Input: part model. Units: mm. Frame: model coordinates. Face numbers are marked on the shaded views. A direction names the side the tool comes from. Give positions to 0.01 mm unless a question says otherwise; leave off trailing zeros. Write each loop counter-clockwise with the first axis right and the second up, starting at its lowest first coordinate (ties: lowest second). Pieces come first, ordered by that corner, then holes.
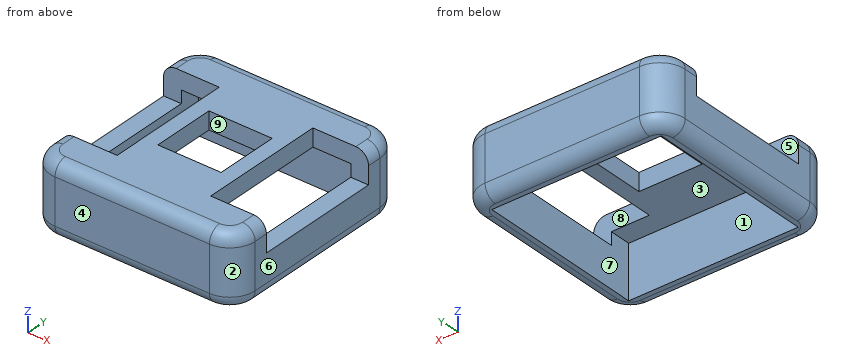
```python
from build123d import *

# Parameters (mm, degrees)
F0_W      = 20.574
F0_H      = 20.574
F1_DEPTH  = 7.112
F2_W      = 17.018
F2_H      = 17.018
F3_DEPTH  = 5.334
F4_R      = 2.54
F5_W      = 5.588
F5_H      = 12.7
F6_DEPTH  = 3.048
F7_W      = 11.176
F7_H      = 12.7
F8_DEPTH  = 3.048
F9_W      = 6.35
F9_H      = 6.35
F10_DEPTH = 1.778
F11_R     = 1.27
F12_R     = 1.27


with BuildPart() as f1:
    # F0 (on Top) → F1 (new body)
    with BuildSketch(Plane.XY):
        Rectangle(F0_W, F0_H)
    extrude(amount=F1_DEPTH)

    # F2 (on face) → F3 (cut)
    with BuildSketch(Plane(origin=(0, 0, 0), x_dir=(1, 0, 0), z_dir=(0, 0, -1))):
        Rectangle(F2_W, F2_H)
    extrude(amount=-F3_DEPTH, mode=Mode.SUBTRACT)

    # F4
    f4_edges = [f1.edges().sort_by_distance(p)[0] for p in [
        (-10.287, -10.287, 3.556),
        (10.287, 10.287, 3.556),
        (10.287, -10.287, 3.556),
        (-10.287, 10.287, 3.556),
    ]]
    fillet(f4_edges, radius=F4_R)

    # F5 (on face) → F6 (cut)
    with BuildSketch(Plane.XY.offset(7.112)):
        with Locations((-7.493, 0)):
            Rectangle(F5_W, F5_H)
    extrude(amount=-F6_DEPTH, mode=Mode.SUBTRACT)

    # F7 (on face) → F8 (cut)
    with BuildSketch(Plane.XY.offset(7.112)):
        with Locations((10.287, 0)):
            Rectangle(F7_W, F7_H)
    extrude(amount=-F8_DEPTH, mode=Mode.SUBTRACT)

    # F9 (on face) → F10 (cut)
    with BuildSketch(Plane.XY.offset(7.112)):
        Rectangle(F9_W, F9_H)
    extrude(amount=-F10_DEPTH, mode=Mode.SUBTRACT)

    # F11
    f11_edges = [f1.edges().sort_by_distance(p)[0] for p in [
        (0, 10.287, 7.112),
        (0, -10.287, 7.112),
    ]]
    fillet(f11_edges, radius=F11_R)

    # F12
    f12_edges = [f1.edges().sort_by_distance(p)[0] for p in [
        (-10.287, 0, 0),
        (0, 10.287, 0),
        (-9.543051, 9.543051, 0),
    ]]
    fillet(f12_edges, radius=F12_R)


solid = f1.part
```
Item 1: Section C-C (x = -7.5). Return loops of the section in (y, z).
Item 2: Section D-D (y = -5.75). Return loops of the section in (x, z).
Item 3: Pin query (flat end, axial travel): pin 1 (2 mm diameter, centred on x = -10, y = 2.5, fed in from +Z); pin 2 (1.5 mm diameter, centred on x = 0, z = 6.5, fed in from +Y); pin 3 (0.5 mm diameter, centred on y = -1, z = 6.5, fed in from +X); pin 4 (2 mm diameter, centred on y = 0.5, z = 6.5, fed in from -X). Return the tip coordinate at first contact, or that it passes through.
Item 4: Mould query, pull axis X, two halves, no side actions, for the marked faces 1, 2, 3 and 4. Classes: +X half, -X half, draft (parallel to the pull), parting line (faces both ways), or undercut.
Item 5: Set-up query: the marked faces 5, 6, 7, 8 and 9. Return all of +Z, -Z, +X, -X, +Y, -Y with unobstructed straight access to the full face (end or side cutting, diameter ignored); none if empty.
Item 6: Ray query, line 1 (Y direction, x = -4, z = 5); line 2 (Y direction, x = -4.75, z = 5.5). Return the intervals inside material, ascending.
Item 7: Section B-B (z = 4.75). Return loops of the section in (x, y), and give its area (3 significant figures).
Item 8: Section A-A (y = 2.5). Return loops of the section in (x, z) (3 decimals), and give its area (3 significant figures).
Solved:
1. outline: (-10.29, 1.27) arc R1.27 ccw to (-9.02, 0) - (-8.51, 0) - (-8.51, 5.33) - (-6.35, 5.33) - (-6.35, 7.11) - (-9.02, 7.11) arc R1.27 ccw to (-10.29, 5.84) - close; (6.35, 5.33) - (8.51, 5.33) - (8.51, 0) - (9.02, 0) arc R1.27 ccw to (10.29, 1.27) - (10.29, 5.84) arc R1.27 ccw to (9.02, 7.11) - (6.35, 7.11) - close
2. outline: (-10.29, 1.27) arc R1.27 ccw to (-9.02, 0) - (-8.51, 0) - (-8.51, 4.06) - (-10.29, 4.06) - close; (-4.7, 5.33) - (4.7, 5.33) - (4.7, 7.11) - (-4.7, 7.11) - close; (8.51, 0) - (9.02, 0) arc R1.27 ccw to (10.29, 1.27) - (10.29, 4.06) - (8.51, 4.06) - close
3. pin 1: stops at z = 4.06
3. pin 2: stops at y = 10.29
3. pin 3: stops at x = 4.7
3. pin 4: stops at x = -4.7
4. face 1: undercut
4. face 2: +X half
4. face 3: undercut
4. face 4: draft
5. face 5: +Z, -X
5. face 6: +Z, -Z, +X, +Y, -Y
5. face 7: -Z
5. face 8: +Z, +X
5. face 9: +Z, -Z
6. line 1: y = -10.29 to -8.51, 8.51 to 10.29
6. line 2: y = -10.29 to -6.35, 6.35 to 10.29
7. outline: (-10.29, -7.75) arc R2.54 ccw to (-7.75, -10.29) - (7.75, -10.29) arc R2.54 ccw to (10.29, -7.75) - (10.29, -6.35) - (8.51, -6.35) - (8.51, -8.51) - (-8.51, -8.51) - (-8.51, -6.35) - (-10.29, -6.35) - close; (-10.29, 6.35) - (-8.51, 6.35) - (-8.51, 8.51) - (8.51, 8.51) - (8.51, 6.35) - (10.29, 6.35) - (10.29, 7.75) arc R2.54 ccw to (7.75, 10.29) - (-7.75, 10.29) arc R2.54 ccw to (-10.29, 7.75) - close
7. area: 83.0 mm2
8. outline: (-10.287, 1.27) arc R1.27 ccw to (-9.017, 0) - (-8.509, 0) - (-8.509, 4.064) - (-10.287, 4.064) - close; (-4.699, 5.334) - (-3.175, 5.334) - (-3.175, 7.112) - (-4.699, 7.112) - close; (3.175, 5.334) - (4.699, 5.334) - (4.699, 7.112) - (3.175, 7.112) - close; (8.509, 0) - (9.017, 0) arc R1.27 ccw to (10.287, 1.27) - (10.287, 4.064) - (8.509, 4.064) - close
8. area: 19.2 mm2
